Verification items for the finished model (mm, model axes). Face numbers are marked on the shaded views. A direction names the side the tool comes from. Coordinates: 2 decimals unless noted, no trailing zeros. Write each loop counter-clockwise with the first axis right and the second up, starting at its lowest first coordinate (ties: lowest second). Pieces come first, ordered by that corner, then holes. Notation, with made-up numbers: M 42.5,73 L 88.5,73 A25 cw 88.5,90 Z; hole C 42,-35 d1. An arc over 180 degrees is marked long. One line per item, written item: value.
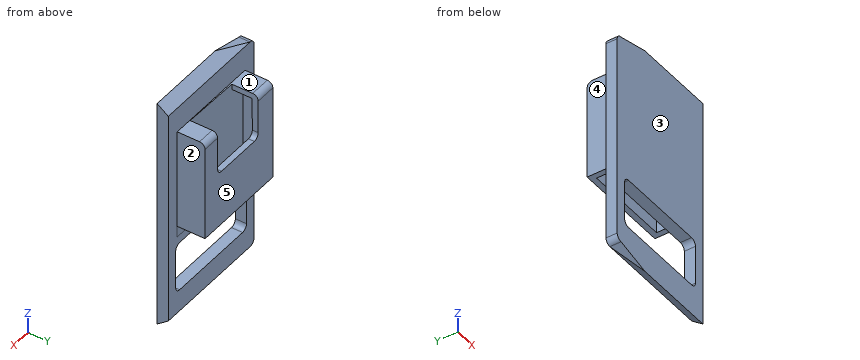
```python
from build123d import *

# Parameters (mm, degrees)
CROQUIS1_W              = 22
CROQUIS1_H              = 39
CROQUIS1_W_2            = 18.17669517928964
CROQUIS1_H_2            = 8.999999999999996
SALIENTE_EXTRUIR1_DEPTH = 2
REDONDEO1_R             = 1
REDONDEO2_R             = 1
SALIENTE_EXTRUIR2_DEPTH = 5
SALIENTE_EXTRUIR4_DEPTH = 15.4
CORTAR_EXTRUIR2_DEPTH   = 8
REDONDEO3_R             = 1
SALIENTE_EXTRUIR5_DEPTH = 20.000000000000004
SALIENTE_EXTRUIR6_DEPTH = 14.9
SALIENTE_EXTRUIR7_DEPTH = 14.9
SALIENTE_EXTRUIR8_DEPTH = 2
CORTAR_EXTRUIR3_DEPTH   = 7
SALIENTE_EXTRUIR9_DEPTH = 2
CORTAR_EXTRUIR4_DEPTH   = 8


with BuildPart() as part:
    # Croquis1 → Saliente-Extruir1 (new body)
    with BuildSketch(Plane(origin=(0, 0, 0), x_dir=(1, 0, 0), z_dir=(0, 1, 0))):
        with Locations((11, 19.5)):
            Rectangle(CROQUIS1_W, CROQUIS1_H)
        with Locations((11.000000000000002, 30.5)):
            Rectangle(CROQUIS1_W_2, CROQUIS1_H_2, mode=Mode.SUBTRACT)
        Polygon((2.2999999999999914, 4.496684869244013), (19.7, 4.496684869244013), (19.7, 22.496684869244014), (18.7, 22.496684869244014), (18.7, 5.496684869244012), (3.299999999999997, 5.496684869244012), (3.299999999999997, 22.49668486924401), (2.2999999999999914, 22.49668486924401), align=None, mode=Mode.SUBTRACT)
    extrude(amount=SALIENTE_EXTRUIR1_DEPTH)

    # Redondeo1
    redondeo1_edges = [part.edges().sort_by_distance(p)[0] for p in [
        (0, 1, -39),
        (0, 1, 0),
    ]]
    fillet(redondeo1_edges, radius=REDONDEO1_R)

    # Redondeo2
    redondeo2_edges = [part.edges().sort_by_distance(p)[0] for p in [
        (1.9116524103551802, 1, -35),
        (1.9116524103551802, 1, -26.000000000000004),
        (20.088347589644822, 1, -26.000000000000004),
        (20.088347589644822, 1, -35),
    ]]
    fillet(redondeo2_edges, radius=REDONDEO2_R)



with BuildPart() as body_2:
    # Croquis8 → Saliente-Extruir2 (new body)
    with BuildSketch(Plane(origin=(0, 2, 0), x_dir=(1, 0, 0), z_dir=(0, 1, 0))):
        Polygon((2.2999999999999914, 22.49668486924401), (3.299999999999997, 22.49668486924401), (3.299999999999997, 5.496684869244012), (18.7, 5.496684869244012), (18.7, 22.496684869244014), (19.7, 22.496684869244014), (19.7, 4.496684869244013), (2.2999999999999914, 4.496684869244013), align=None)
    extrude(amount=SALIENTE_EXTRUIR2_DEPTH)

    # Croquis3D1 → Saliente-Extruir4 (add)
    with BuildSketch(Plane(origin=(18.7, 6.007354442998164, -22.496684869244014), x_dir=(0, 0.058291627055225136, 0.9982995974231657), z_dir=(1, 0, 0))):
        Polygon((0, 0), (16.964879958528087, 1.097364583913252), (17.028956080800597, 0), (0.05786292460677727, -0.9909576599388273), align=None)
    extrude(amount=-SALIENTE_EXTRUIR4_DEPTH)

    # Croquis3D2 → Cortar-Extruir2 (cut)
    with BuildSketch(Plane(origin=(6.0546274348603735, 7, -4.496684869244013), x_dir=(0.9015563394045935, -0.4326617233814304, 0), z_dir=(0, 0, -1))):
        Polygon((0, 0), (2.1633086169071523, 4.507781697022968), (11.556372403185868, 0), (9.393063786278717, -4.507781697022968), align=None)
    extrude(amount=CORTAR_EXTRUIR2_DEPTH, mode=Mode.SUBTRACT)

    # Redondeo3
    redondeo3_edges = [body_2.edges().sort_by_distance(p)[0] for p in [
        (6.0546274348603735, 6.4723277606850065, -12.496684869244014),
        (16.47334823547289, 6.4723277606850065, -12.496684869244014),
        (18.086674117736443, 7, -4.496684869244013),
        (4.177313717430181, 7, -4.496684869244013),
    ]]
    fillet(redondeo3_edges, radius=REDONDEO3_R)


with BuildPart() as part_1:
    add(part.part)

    add(body_2.part)  # Saliente-Extruir5 merges body 2
    # Croquis15 → Saliente-Extruir5 (add)
    with BuildSketch(Plane(origin=(0, 0, -4.496684869244013), x_dir=(-1, 0, 0), z_dir=(0, 0, -1))):
        Polygon((-19.7, 2), (-19.7, 0), (-2.2999999999999914, 0), (-2.2999999999999914, 2.336560166952495), align=None)
    extrude(amount=SALIENTE_EXTRUIR5_DEPTH)

    # Croquis16 → Saliente-Extruir6 (add)
    with BuildSketch(Plane(origin=(22, 0, 0), x_dir=(0, 0, -1), z_dir=(1, 0, 0))):
        Polygon((0, 0), (-1.5, -1.8e-16), (0, 2), align=None)
    extrude(amount=-SALIENTE_EXTRUIR6_DEPTH)

    # Croquis17 → Saliente-Extruir7 (add)
    with BuildSketch(Plane(origin=(22, 0, 0), x_dir=(0, 0, -1), z_dir=(1, 0, 0))):
        Polygon((39, 0), (40.5, 0), (39, 2), align=None)
    extrude(amount=-SALIENTE_EXTRUIR7_DEPTH)

    # Croquis18 → Saliente-Extruir8 (add)
    with BuildSketch(Plane.XZ):
        Polygon((7.099999999999999, 1.5), (0.9999999999999966, 0), (7.099999999999999, 0), align=None)
    extrude(amount=-SALIENTE_EXTRUIR8_DEPTH)

    # Croquis20 → Cortar-Extruir3 (cut)
    with BuildSketch(Plane(origin=(7.099999999999999, 0, 0), x_dir=(0, 0, -1), z_dir=(1, 0, 0))):
        Polygon((0, 2), (-1.5, 2), (-1.5, 0), align=None)
    extrude(amount=-CORTAR_EXTRUIR3_DEPTH, mode=Mode.SUBTRACT)

    # Croquis22 → Saliente-Extruir9 (add)
    with BuildSketch(Plane(origin=(0, 2, 0), x_dir=(1, 0, 0), z_dir=(0, 1, 0))):
        Polygon((7.099999999999999, 40.5), (7.099999999999999, 39), (1, 39), align=None)
    extrude(amount=-SALIENTE_EXTRUIR9_DEPTH)

    # Croquis23 → Cortar-Extruir4 (cut)
    with BuildSketch(Plane(origin=(7.099999999999999, 0, 0), x_dir=(0, 0, -1), z_dir=(1, 0, 0))):
        Polygon((40.5, 0), (39, 2), (40.5, 2), align=None)
    extrude(amount=-CORTAR_EXTRUIR4_DEPTH, mode=Mode.SUBTRACT)


solid = part_1.part
```
Item 1: Access from +Z, -Z, +X, -X, +Y, -Y to the whole of each face (thin tool, end or side, straight path). Record for the marked faces 1, 2, 3, 4 and 5.
The answers:
face 1: +Z, +X, -X, +Y
face 2: +Z, -Z, +X, +Y
face 3: +Z, -Z, +X, -X, -Y
face 4: +Z, -Z, -X, +Y
face 5: +Z, -Z, +X, -X, +Y
Item 2: Go/stop test with flat-tipped pins: P1, Ø1.8, axis at y = 5, z = -18, coming from the +X side; P2, Ø2.5, axis at y = 3.5, z = -7, coming from the -X side; P3, Ø0.5, axis at x = 13, y = 6.5, coming from the +Z side; P4, Ø2, axis at x = 12.5, y = 4.5, coming from the -Z side. Record where each tip stops, or that it passes through.
The answers:
P1: stops at x = 19.7
P2: stops at x = 2.3
P3: stops at z = -12.5
P4: passes through
Item 3: Cross-section at D-D, the plane z = -14. Enter the section's corners in (x, y).
The answers:
outline: M 0,0 L 22,0 L 22,2 L 19.7,2 L 19.7,7 L 2.3,7 L 2.3,2 L 0,2 Z; hole M 3.3,2.32 L 18.7,2.02 L 18.7,5.95 L 3.3,5.95 Z
Item 4: Cross-section at A-A, the plane y = 4. Enter the section's corners in (x, z).
The answers:
outline: M 2.3,-22.5 L 3.3,-22.5 L 3.3,-5.5 L 6.05,-5.5 L 6.05,-4.5 L 2.3,-4.5 Z; M 16.47,-5.5 L 18.7,-5.5 L 18.7,-22.5 L 19.7,-22.5 L 19.7,-4.5 L 16.47,-4.5 Z
Item 5: Cross-section at B-B, the plane x = 10.5. Enter the section's corners in (y, z).
The answers:
outline: M 0,-40.5 L 2,-39 L 2,-35 L 0,-35 Z; M 0,-26 L 2,-26 L 2,-24.5 L 2.18,-24.5 L 2.18,-4.5 L 2,-4.5 L 2,0 L 0,1.5 Z; M 5.94,-12.5 L 6.01,-22.5 L 7,-22.5 L 7,-12.5 Z
Item 6: Scan lines: line 1 (X direction, y = 5.5, z = -5); line 2 (Y direction, x = 18.5, z = -7); line 3 (Y direction, x = 3.5, z = -22). Record each from-to range of solid material in increasing order.
The answers:
line 1: x = 2.3 to 6.05, 16.47 to 19.7
line 2: y = 0 to 2.02, 5.91 to 7
line 3: y = 0 to 2.31, 6 to 7
Item 7: Cross-section at C-C, the plane z = -34.5. Enter the section's corners in (x, y).
The answers:
outline: M 0,0 L 2.05,0 L 2.05,2 L 0,2 Z; M 19.95,0 L 22,0 L 22,2 L 19.95,2 Z
